Input: part model. Units: mm. Frame: model coordinates. A direction names the side the tool comes from. Coordinates: 2 decimals unless noted, no trailing zeros. Loops run counter-clockwise (first coordinate to the right, second up) from the corner with the lowest first, then second, coordinate; pieces in that order, holes last.
Item 1: Ray query, line 1 along Z through (x, y) = (12, 25); line 2 along Y through (x, z) = (2.5, -5.5); line 3 along Y through (x, z) = (8.5, 3.5). Return the intervals inside material, ascending.
Item 2: Reachability of faces 4 (the flat face through (1.57, -16.9, -6.23)), 5 (the flat face through (10, 20.25, 7)), 6 (the flat face through (6.75, 24, 10)) from +Z, -Z, +X, -X, +Y, -Y: full face, straight path, thin tool, end or side. Return the list, or none.
Item 3: Section D-D on x = 13. Return loops of the section in (y, z).
Item 4: Section A-A on y = -22. Return loops of the section in (x, z), and give its area (3 significant figures).
Item 5: Section B-B on x = 23. Return loops of the section in (y, z).
Item 6: Pull-direction query (X, two-part tool) for faces 1 (the flat face through (-4, 12.05, 5)), 2 (the flat face through (20, -24, -2.9)), 3 (the cylindrical face through (-5.32, -26.75, 3.32)); classes: released by +X, released by -X, zero draft, split by the parting line, or undercut.
Item 7: Contact query for flat-ended pins moving along their axis: P1, Ø2.5, axis at y = -24.25, z = 0, coming from the +X side; P2, Ø2, axis at y = 10, z = 5.5, coming from the +X side; P3, Ø5, axis at x = 0.86, y = 14.14, coming from the +Z side; P4, Ø3, axis at y = -24.25, z = 10, coming from the -X side. Output: stop coordinate, or through.
```python
from build123d import *

# Parameters (mm, degrees)
PAD004_DEPTH    = 5
PAD003_DEPTH    = 20
POCKET018_DEPTH = 20
SKETCH024_R     = 16.5
POCKET017_DEPTH = 5
SKETCH017_R     = 1.6
POCKET014_DEPTH = 5
POCKET019_DEPTH = 2.5
SKETCH020_W     = 3
SKETCH020_H     = 5.8
POCKET013_DEPTH = 56.5
SKETCH022_R     = 1.6
POCKET020_DEPTH = 18
SKETCH019_R     = 0.95
POCKET016_DEPTH = 3
POCKET015_DEPTH = 1.5
PAD_DEPTH       = 5
FILLET_R        = 2.99
POCKET_DEPTH    = 6.8
FILLET001_R     = 0.4
POCKET021_DEPTH = 13


with BuildPart() as part:
    # Sketch023 → Pad004 (new body)
    with BuildSketch(Plane.XY):
        with BuildLine():
            Line((-16.75, 28.25), (16.75, 28.25))
            ThreePointArc((21.75, 23.25), (20.285534, 26.785534), (16.75, 28.25))
            Line((21.75, 23.25), (21.75, -23.25))
            ThreePointArc((16.75, -28.25), (20.285534, -26.785534), (21.75, -23.25))
            Line((16.75, -28.25), (-16.75, -28.25))
            ThreePointArc((-21.75, -23.25), (-20.285534, -26.785534), (-16.75, -28.25))
            Line((-21.75, -23.25), (-21.75, 23.25))
            ThreePointArc((-16.75, 28.25), (-20.285534, 26.785534), (-21.75, 23.25))
        make_face()
    extrude(amount=PAD004_DEPTH)

    # Pad004 Face10 → Pad003 (add)
    with BuildSketch(Plane(origin=(0, 0, 5), x_dir=(0, 1, 0), z_dir=(0, 0, 1))):
        with BuildLine():
            Line((23.25, 21.75), (-23.25, 21.75))
            ThreePointArc((-23.25, 21.75), (-26.785534, 20.285534), (-28.25, 16.75))
            Line((-28.25, 16.75), (-28.25, -16.75))
            ThreePointArc((-28.25, -16.75), (-26.785534, -20.285534), (-23.25, -21.75))
            Line((-23.25, -21.75), (23.25, -21.75))
            ThreePointArc((23.25, -21.75), (26.785534, -20.285534), (28.25, -16.75))
            Line((28.25, -16.75), (28.25, 16.75))
            ThreePointArc((28.25, 16.75), (26.785534, 20.285534), (23.25, 21.75))
        make_face()
    extrude(amount=PAD003_DEPTH)

    # Sketch026 (on Face13 of Pad003) → Pocket018 (cut)
    with BuildSketch(Plane.XY.offset(25)):
        Polygon((9.75, 28.25), (9.75, 20.25), (-18.75, 20.25), (-18.75, -20.25), (9.75, -20.25), (9.75, -28.25), (21.75, -28.25), (21.75, 28.25), align=None)
    extrude(amount=-POCKET018_DEPTH, mode=Mode.SUBTRACT)

    # Sketch024 (on Face14 of Pocket018) → Pocket017 (cut)
    with BuildSketch(Plane.XY.offset(5)):
        Circle(SKETCH024_R)
    extrude(amount=-POCKET017_DEPTH, mode=Mode.SUBTRACT)

    # Sketch017 (on Face15 of Pocket017) → Pocket014 (cut)
    with BuildSketch(Plane.XY.offset(5)):
        with Locations((-14.142136, 14.142136)):
            Circle(SKETCH017_R)
        with Locations((14.142136, 14.142136)):
            Circle(SKETCH017_R)
        with Locations((14.142136, -14.142136)):
            Circle(SKETCH017_R)
        with Locations((-14.142136, -14.142136)):
            Circle(SKETCH017_R)
    extrude(amount=-POCKET014_DEPTH, mode=Mode.SUBTRACT)

    # Sketch021 (on Face19 of Pocket014) → Pocket019 (cut)
    with BuildSketch(Plane.XY.offset(5)):
        Polygon((-11.81512, 16.469151), (-14.993882, 17.320898), (-17.320898, 14.993882), (-16.469151, 11.81512), (-13.290389, 10.963374), (-10.963374, 13.290389), align=None)
        Polygon((14.993882, 17.320898), (11.81512, 16.469151), (10.963374, 13.290389), (13.290389, 10.963374), (16.469151, 11.81512), (17.320898, 14.993882), align=None)
        Polygon((-13.290389, -10.963374), (-16.469151, -11.81512), (-17.320898, -14.993882), (-14.993882, -17.320898), (-11.81512, -16.469151), (-10.963374, -13.290389), align=None)
        Polygon((16.469151, -11.81512), (13.290389, -10.963374), (10.963374, -13.290389), (11.81512, -16.469151), (14.993882, -17.320898), (17.320898, -14.993882), align=None)
    extrude(amount=-POCKET019_DEPTH, mode=Mode.SUBTRACT)

    # Sketch020 (on Face20 of Pocket019) → Pocket013 (cut)
    with BuildSketch(Plane.XZ.offset(28.25)):
        with Locations((5.25, 20)):
            Rectangle(SKETCH020_W, SKETCH020_H)
        with Locations((5.25, 10)):
            Rectangle(SKETCH020_W, SKETCH020_H)
    extrude(amount=-POCKET013_DEPTH, mode=Mode.SUBTRACT)

    # Sketch022 (on Face26 of Pocket013) → Pocket020 (cut)
    with BuildSketch(Plane.YZ.offset(9.75)):
        with Locations((-24.25, 20)):
            Circle(SKETCH022_R)
        with Locations((-24.25, 10)):
            Circle(SKETCH022_R)
        with Locations((24.25, 20)):
            Circle(SKETCH022_R)
        with Locations((24.25, 10)):
            Circle(SKETCH022_R)
    extrude(amount=-POCKET020_DEPTH, mode=Mode.SUBTRACT)

    # Sketch019 (on Face28 of Pocket020) → Pocket016 (cut)
    with BuildSketch(Plane.YZ.offset(-18.75)):
        with Locations((10, 15)):
            Circle(SKETCH019_R)
    extrude(amount=-POCKET016_DEPTH, mode=Mode.SUBTRACT)

    # Sketch018 (on Face29 of Pocket016) → Pocket015 (cut)
    with BuildSketch(Plane.YZ.offset(-18.75)):
        Polygon((12.05, 13.816432), (12.05, 16.183568), (10, 17.367136), (7.95, 16.183568), (7.95, 13.816432), (10, 12.632864), align=None)
    extrude(amount=-POCKET015_DEPTH, mode=Mode.SUBTRACT)

    # Pocket015 Face18 → Pad (add)
    with BuildSketch(Plane(origin=(-8.560893, 0, 25), x_dir=(0, 1, 0), z_dir=(0, 0, 1))):
        with BuildLine():
            ThreePointArc((-23.25, 13.189107), (-26.785534, 11.724641), (-28.25, 8.189107))
            Line((-28.25, 8.189107), (-28.25, -18.310893))
            Line((-28.25, -18.310893), (-20.25, -18.310893))
            Line((-20.25, -18.310893), (-20.25, 10.189107))
            Line((-20.25, 10.189107), (20.25, 10.189107))
            Line((20.25, 10.189107), (20.25, -18.310893))
            Line((20.25, -18.310893), (28.25, -18.310893))
            Line((28.25, -18.310893), (28.25, 8.189107))
            ThreePointArc((28.25, 8.189107), (26.785534, 11.724641), (23.25, 13.189107))
            Line((23.25, 13.189107), (-23.25, 13.189107))
        make_face()
    extrude(amount=PAD_DEPTH)

    # Fillet
    fillet_edges = [part.edges().sort_by_distance(p)[0] for p in [
        (-3.5, 28.25, 30),
    ]]
    fillet(fillet_edges, radius=FILLET_R)

    # Sketch (on Face40 of Fillet) → Pocket (cut)
    with BuildSketch(Plane.XZ.offset(-20.25)):
        with BuildLine():
            ThreePointArc((-14.25, 11.5), (-11.75, 9), (-9.25, 11.5))
            Line((-9.25, 30), (-9.25, 11.5))
            Line((-14.25, 30), (-9.25, 30))
            Line((-14.25, 11.5), (-14.25, 30))
        make_face()
    extrude(amount=-POCKET_DEPTH, mode=Mode.SUBTRACT)

    # Fillet001
    fillet001_edges = [part.edges().sort_by_distance(p)[0] for p in [
        (-11.75, 27.05, 29.404995),
        (-14.25, 22.755, 30),
        (-9.25, 22.755, 30),
        (-4.5, -20.25, 30),
        (-16.5, 20.25, 30),
        (0.25, 20.25, 30),
        (9.75, -22.755, 30),
        (9.75, 22.755, 30),
    ]]
    fillet(fillet001_edges, radius=FILLET001_R)

    # Sketch032 → Pocket021 (cut)
    with BuildSketch(Plane.YZ.offset(5.75)):
        Polygon((28.25, 24.089384), (28.25, 27.338749), (20.25, 28.749365), (20.25, 25.5), align=None)
    extrude(amount=-POCKET021_DEPTH, mode=Mode.SUBTRACT)


with BuildPart() as part_1:
    # Body005 placement: moved
    add(part.part.moved(Location((15, 0, -10))))


solid = part_1.part
```
Results found:
1. line 1: z = -10 to -1.41, 1.41 to 8.59, 11.41 to 14.66, 17.91 to 20
1. line 2: y = -28.25 to -16.65, -11.75 to -10.77, 10.77 to 11.75, 16.65 to 28.25
1. line 3: y = -28.25 to -20.25, 20.25 to 28.25
2. face 4: +Z
2. face 5: +Z, +X
2. face 6: +X
3. outline: (-28.25, -10) - (-16.38, -10) - (-16.38, -5) - (-20.25, -5) - (-20.25, 19.6) arc R0.4 ccw to (-20.65, 20) - (-25.26, 20) arc R2.99 ccw to (-28.25, 17.01) - close; (16.38, -10) - (28.25, -10) - (28.25, 14.09) - (20.25, 15.5) - (20.25, -5) - (16.38, -5) - close; (20.25, 18.75) - (28.23, 17.34) arc R2.99 ccw to (25.26, 20) - (20.65, 20) arc R0.4 ccw to (20.25, 19.6) - close; hole circle Ø3.2 at (-24.25, 0); hole circle Ø3.2 at (-24.25, 10); hole circle Ø3.2 at (24.25, 0); hole circle Ø3.2 at (24.25, 10)
4. outline: (-6.75, -10) - (36.75, -10) - (36.75, -5) - (24.75, -5) - (24.75, 19.6) arc R0.4 ccw to (24.35, 20) - (-3.76, 20) arc R2.99 ccw to (-6.75, 17.01) - close; hole (18.75, -2.9) - (21.75, -2.9) - (21.75, 2.9) - (18.75, 2.9) - close; hole (18.75, 7.1) - (21.75, 7.1) - (21.75, 12.9) - (18.75, 12.9) - close
4. area: 968 mm2
5. outline: (-28.25, -10) - (-14.43, -10) - (-14.43, -5) - (-20.25, -5) - (-20.25, 19.6) arc R0.4 ccw to (-20.65, 20) - (-25.26, 20) arc R2.99 ccw to (-28.25, 17.01) - close; (14.43, -10) - (28.25, -10) - (28.25, 17.01) arc R2.99 ccw to (25.26, 20) - (20.65, 20) arc R0.4 ccw to (20.25, 19.6) - (20.25, -5) - (14.43, -5) - close; hole circle Ø3.2 at (-24.25, 0); hole circle Ø3.2 at (-24.25, 10); hole circle Ø3.2 at (24.25, 0); hole circle Ø3.2 at (24.25, 10)
6. face 1: zero draft
6. face 2: undercut
6. face 3: released by -X
7. P1: stops at x = 6.75
7. P2: stops at x = -5.25
7. P3: stops at z = -7.5
7. P4: stops at x = -6.75
